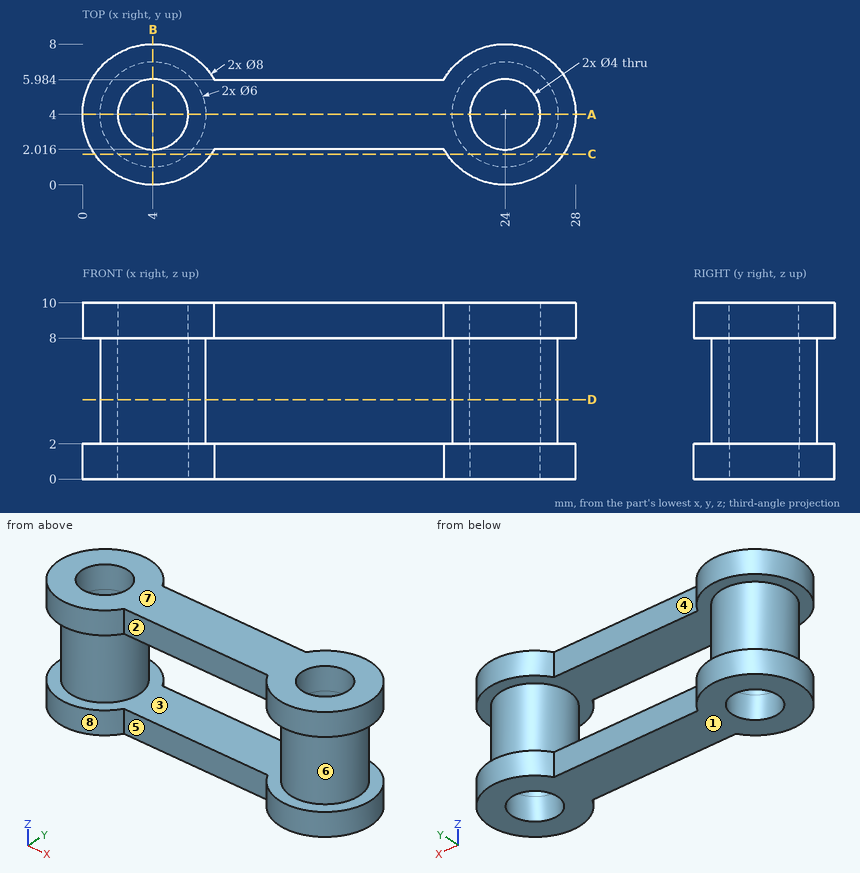
For this review, use the dimensioned drawing (mm, ordinates from the lowest corner) and the shaded views. A direction names the side the tool comes from. Coordinates: 2 decimals unless noted, no trailing zeros. Loops run counter-clockwise (first coordinate to the right, second up) from the corner with the lowest first, then second, coordinate; pieces in that order, holes last. Notation, with made-up numbers: (59.5, -14.75) -> (85.5, -14.75) arc R27 ccw to (85.5, 8.25) -> close; hole circle Ø1 at (20, 16.25). An arc over 180 degrees is marked (long way). Use a Markdown table: item, result. Add a question column.
1. Add section B-B on x = 4. Write out the cut boundary in (y, z), plus the area to 3 significant figures.
2. Add section C-C on y = 1.75. Write out the cut boundary in (x, z), plus the area to 3 significant figures.
3. Add section A-A on y = 4. Write out the cut boundary in (x, z), plus the area to 3 significant figures.
4. Machinability: for the marked faces 4, 5, 6, 7 and 8, which of the approach directions +Z, -Z, +X, -X, +Y, -Y give a long, thin tool a straight path to every point of the face, cutting with its end or side? Answer none if there is none.
5. Draft analysis for pull direction Z (two halves, no side actions). For the marked faces 1, 2 and 3, state which applies: pulls with the +Z half, pulls with the -Z half, needs draft (parallel to the pull), parting line crosses it, or undercut.
6. Add section D-D on z = 4.5. Write out the cut boundary in (x, y).
7. To check wall thickness, follow line 1 (Y direction, x = 24, z = 6.4); line 2 (Z direction, x = 19.5, y = 4.5); line 3 (Y direction, x = 4, z = 1.45). State the ranges of each line that lie inside material, in increasing order.
8. Clearance check with flat-ended pins moving along their axes: pin 1 Ø0.6 at (x, z) = (13.5, 1.5) entering from -Y; pin 2 Ø1 at (x, z) = (14.5, 9.5) entering from +Y; pin 3 Ø3 at (x, z) = (6, 2) entering from -Y. State where each tip first meets the part, or that it passes through.
Returned:
| question | item | result |
|---|---|---|
| 1 | outline | (0, 0) -> (2, 0) -> (2, 10) -> (0, 10) -> (0, 8) -> (1, 8) -> (1, 2) -> (0, 2) -> close; (6, 0) -> (8, 0) -> (8, 2) -> (7, 2) -> (7, 8) -> (8, 8) -> (8, 10) -> (6, 10) -> close |
| 1 | area | 28.0 mm² |
| 2 | outline | (0.69, 0) -> (7.31, 0) -> (7.31, 2) -> (5.98, 2) -> (5.98, 8) -> (7.31, 8) -> (7.31, 10) -> (0.69, 10) -> (0.69, 8) -> (2.02, 8) -> (2.02, 2) -> (0.69, 2) -> close; (20.69, 0) -> (27.31, 0) -> (27.31, 2) -> (25.98, 2) -> (25.98, 8) -> (27.31, 8) -> (27.31, 10) -> (20.69, 10) -> (20.69, 8) -> (22.02, 8) -> (22.02, 2) -> (20.69, 2) -> close |
| 2 | area | 101 mm² |
| 3 | outline | (0, 0) -> (2, 0) -> (2, 10) -> (0, 10) -> (0, 8) -> (1, 8) -> (1, 2) -> (0, 2) -> close; (6, 0) -> (22, 0) -> (22, 10) -> (6, 10) -> close; (26, 0) -> (28, 0) -> (28, 2) -> (27, 2) -> (27, 8) -> (28, 8) -> (28, 10) -> (26, 10) -> close; hole (7, 2) -> (21, 2) -> (21, 8) -> (7, 8) -> close |
| 3 | area | 104 mm² |
| 4 | face 4 | +Z, -Z, +Y |
| 4 | face 5 | +Z, -Z, -Y |
| 4 | face 6 | none |
| 4 | face 7 | +Z, +X, -X, +Y, -Y |
| 4 | face 8 | +Z, -Z |
| 5 | face 1 | pulls with the -Z half |
| 5 | face 2 | needs draft |
| 5 | face 3 | undercut |
| 6 | outline | circle Ø6 at (4, 4); circle Ø6 at (24, 4); hole circle Ø4 at (4, 4); hole circle Ø4 at (24, 4) |
| 7 | line 1 | y = 1 to 2, 6 to 7 |
| 7 | line 2 | z = 0 to 2, 8 to 10 |
| 7 | line 3 | y = 0 to 2, 6 to 8 |
| 8 | pin 1 | stops at y = 2.02 |
| 8 | pin 2 | stops at y = 5.98 |
| 8 | pin 3 | stops at y = 0.03 |
